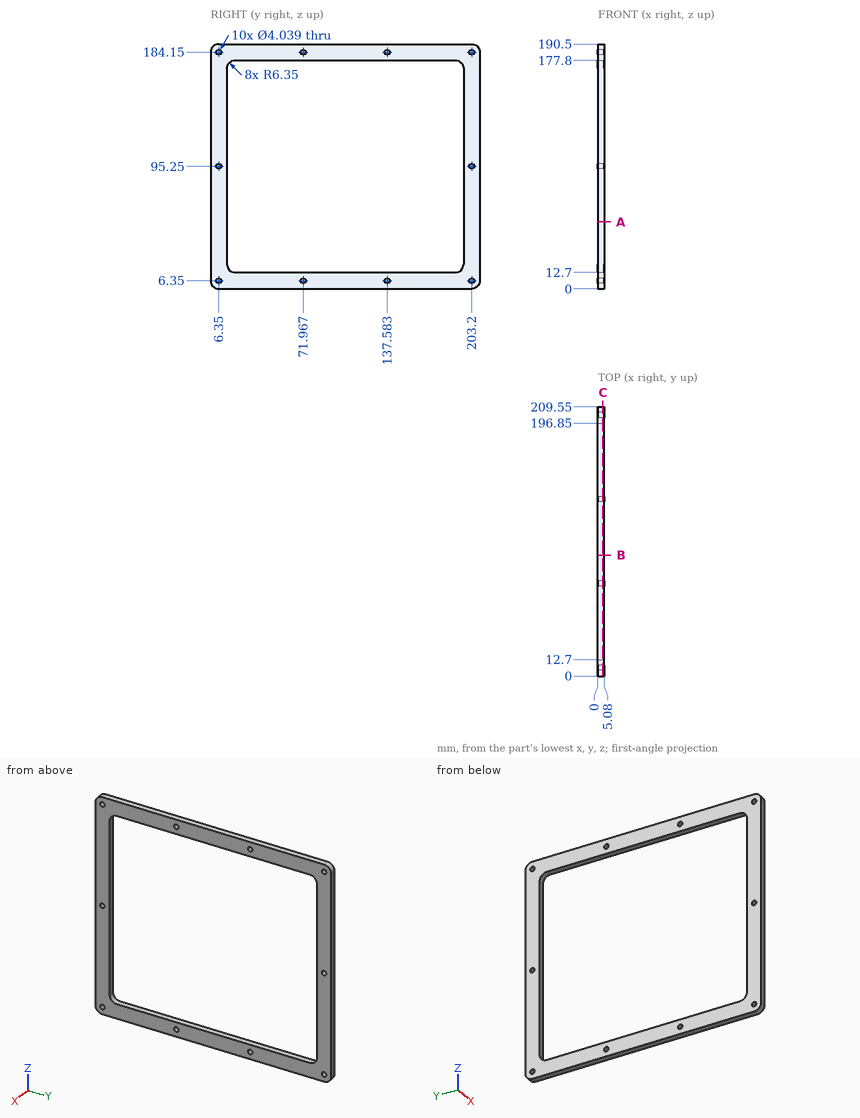
Source: three-view drawing plus pictorial views. Frame: mm from the lowest corner of the part. Give positions to 0.01 mm unless a question says otherwise; leave off trailing zeros. Order: outer loops, then holes, each group sorted by start corner. A loop starts at its lowest first (then second) coordinate and runs counter-clockwise, first axis right, second up. Notation, with made-up numbers: (72, 21.5) - (131, 21.5) arc R37 ccw to (131, 57.5) - close; hole circle Ø7 at (-28.75, -18). An arc over 180 degrees is marked (long way). Answer as a JSON object with one key per item and string values. Group by question number.
Q1. Line query: probe 1 along Y at (x, z) = (1.2, 184.15); probe 2 along Y at (x, z) = (4.6, 113.5); probe 3 along Z at (x, y) = (4.45, 126.5). Output: solid intervals per line, ascending.
Q2. First-contact query: pin 1 Ø3 at (x, z) = (0.5, 137.5) entering from -Y; pin 2 Ø3 at (y, z) = (203.2, 95.25) entering from +X. Flat tips, straight axial feed; report the tip coordinate or a pass-through.
Q3. Cut plane A-A, the plane z = 52. Output: boundary loops of the cut face in (x, y), then the cut area to 3 significant figures.
Q4. Cut plane C-C, the plane x = 3.9. Count the separate pieces of the cut face and the enclosed holes in it, then the cut area to 3 significant figures.
Q5. Cut plane B-B, the plane y = 94. Output: boundary loops of the cut face in (x, z), then the cut area to 3 significant figures.
Results:
{
 "1": {"probe 1": "0 to 4.33, 8.37 to 69.95, 73.99 to 135.56, 139.6 to 201.18, 205.22 to 209.55", "probe 2": "0 to 12.7, 196.85 to 209.55", "probe 3": "0 to 12.7, 177.8 to 190.5"},
 "2": {"pin 1": "y = 0", "pin 2": "through"},
 "3": {"outline": "(0, 0) - (5.08, 0) - (5.08, 12.7) - (0, 12.7) - close; (0, 196.85) - (5.08, 196.85) - (5.08, 209.55) - (0, 209.55) - close", "area": "129 mm^2"},
 "4": {"separate pieces": "1", "enclosed holes": "11", "area": "9,390 mm^2"},
 "5": {"outline": "(0, 0) - (5.08, 0) - (5.08, 12.7) - (0, 12.7) - close; (0, 177.8) - (5.08, 177.8) - (5.08, 190.5) - (0, 190.5) - close", "area": "129 mm^2"}
}
